For this review, take the finished solid that the model builds, in its own axes (mm). Face numbers are marked on the shaded views. A direction names the side the tool comes from. Give positions to 0.01 mm unless a question says otherwise; leave off trailing zeros. Write each loop counter-clockwise with the first axis right and the second up, starting at its lowest first coordinate (ties: lowest second). Pieces come first, ordered by that corner, then holes.
1) For P1, Ø3, axis at y = 3, z = 9, coming from the -X side; P2, Ø3, axis at x = 0, z = 8.03, coming from the +Y side, all flat-tipped, find the tip position at first contact; note any pin that passes through.
2) Wall thickness on line 1 along X through (y, z) = (1.1, 13); line 2 along X through (y, z) = (1.2, 14.5); line 3 along Y through (x, z) = (-1.5, 1.5): over which ranges is each line inside the solid? List them lowest first.
3) We need section B-B on y = 1.3. Give the number of separate pieces and of enclosed holes in the cut face, and give its area (3 significant figures).
4) We need section A-A on z = 6. Give the boundary of the cut face in (x, y), and give its area (3 significant figures).
5) Draft analysis for pull direction Z (two halves, no side actions). For the marked faces 6, 7, 8 and 9, state which applies: pulls with the +Z half, pulls with the -Z half, needs draft (parallel to the pull), parting line crosses it, or undercut.
6) Machinability: for the marked faces 1, 2, 3, 4 and 5, which of the approach directions +Z, -Z, +X, -X, +Y, -Y give a long, thin tool a straight path to every point of the face, cutting with its end or side? Answer none if there is none.
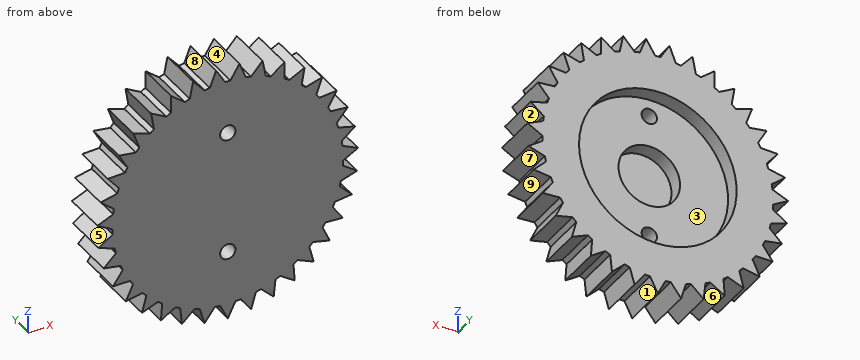
from build123d import *

# Parameters (mm, degrees)
SKETCH_1_R          = 15
EXTRUDE_1_DEPTH     = 6
EXTRUDE_2_DEPTH     = 6
SKETCH_3_R          = 1
CUT_EXTRUDE_1_DEPTH = 6
SKETCH_4_R          = 10.25
CUT_EXTRUDE_2_DEPTH = 2
SKETCH_5_R          = 4
CUT_EXTRUDE_3_DEPTH = 2


with BuildPart() as part:
    # 草图1 → 凸台-拉伸1 (new body)
    with BuildSketch(Plane(origin=(0, 0, 0), x_dir=(1, 0, 0), z_dir=(0, 1, 0))):
        Circle(SKETCH_1_R)
    extrude(amount=EXTRUDE_1_DEPTH)

    # 草图2 → 凸台-拉伸2 (add)
    with BuildSketch(Plane(origin=(0, 6, 0), x_dir=(1, 0, 0), z_dir=(0, 1, 0))):
        Polygon((0, 16.966629547), (-1, 14.966629547), (-1, 14.940773363), (1, 14.940773363), (1, 14.966629547), align=None)
        Polygon((3.656324486, 14.547552758), (3.029508687, 16.69396883), (1.688465309, 14.904666548), (1.683848509, 14.879225883), (3.651707686, 14.522112094), align=None)
        Polygon((6.195131695, 13.660905654), (5.961646472, 15.884750219), (4.322661954, 14.363655302), (4.313576741, 14.339447841), (6.186046483, 13.636698193), align=None)
        Polygon((8.534822274, 12.335185802), (8.702172035, 14.564982666), (6.817924686, 13.360984356), (6.804663068, 13.338788146), (8.521560655, 12.312989592), align=None)
        Polygon((10.600196642, 10.613002928), (11.163002628, 12.777084586), (9.09405371, 11.92888038), (9.077041925, 11.909408826), (10.583184857, 10.593531374), align=None)
        Polygon((12.324871968, 8.549709408), (13.265045131, 10.578520495), (11.077892365, 10.113372373), (11.057677186, 10.097251306), (12.30465679, 8.533588341), align=None)
        Polygon((13.653415769, 6.211621193), (14.94073817, 8.03995405), (12.705678444, 7.972812257), (12.682909604, 7.960559822), (13.630646929, 6.199368758), align=None)
        Polygon((14.543127552, 3.673886362), (16.13622359, 5.242976867), (13.925093563, 5.575999395), (13.900502871, 5.568009395), (14.51853686, 3.665896362), align=None)
        Polygon((14.96541125, 1.018069801), (16.813077508, 2.277486094), (14.696944718, 2.999969324), (14.671322539, 2.996498564), (14.939789071, 1.014599041), align=None)
        Polygon((14.906694317, -1.670468362), (16.94954528, -0.761204956), (14.996423977, 0.327517771), (14.970593829, 0.328677804), (14.880864168, -1.669308329), align=None)
        Polygon((14.368863963, -4.305316297), (16.541240721, -3.775430253), (14.813905831, -2.355460473), (14.788697915, -2.349706931), (14.343656047, -4.299562755), align=None)
        Polygon((13.369206498, -6.801787824), (15.601287075, -6.668310115), (14.155256562, -4.962732279), (14.131481082, -4.952570151), (13.345431019, -6.791625697), align=None)
        Polygon((11.939851737, -9.079644294), (14.159895226, -9.346865003), (13.0416457, -7.410497786), (13.02006682, -7.396253693), (11.918272857, -9.0654002), align=None)
        Polygon((10.126740316, -11.065673525), (12.263392693, -11.725003959), (11.508865614, -9.620083797), (11.490176897, -9.602215554), (10.1080516, -11.047805282), align=None)
        Polygon((7.98814713, -12.696042904), (9.972734629, -13.726291641), (9.606181119, -11.5204724), (9.590983235, -11.499554308), (7.972949246, -12.675124812), align=None)
        Polygon((5.592808322, -13.918351018), (7.361544668, -15.286405015), (7.394746058, -13.05058354), (7.38352748, -13.027287923), (5.581589744, -13.895055402), align=None)
        Polygon((3.017712053, -14.693311879), (4.513748605, -16.355200755), (4.945637774, -14.161238188), (4.938759077, -14.136313787), (3.010833355, -14.668387478), align=None)
        Polygon((0.345624035, -14.996017606), (1.520876947, -16.898326885), (2.337572623, -14.816738988), (2.335254893, -14.790986893), (0.343306305, -14.970265511), align=None)
        Polygon((-2.337572623, -14.816738988), (-1.520876947, -16.898326885), (-0.345624035, -14.996017606), (-0.343306305, -14.970265511), (-2.335254893, -14.790986893), align=None)
        Polygon((-4.945637774, -14.161238188), (-4.513748605, -16.355200755), (-3.017712053, -14.693311879), (-3.010833355, -14.668387478), (-4.938759077, -14.136313787), align=None)
        Polygon((-7.394746058, -13.05058354), (-7.361544668, -15.286405015), (-5.592808322, -13.918351018), (-5.581589744, -13.895055402), (-7.38352748, -13.027287923), align=None)
        Polygon((-9.606181119, -11.5204724), (-9.972734629, -13.726291641), (-7.98814713, -12.696042904), (-7.972949246, -12.675124812), (-9.590983235, -11.499554308), align=None)
        Polygon((-11.508865614, -9.620083797), (-12.263392693, -11.725003959), (-10.126740316, -11.065673525), (-10.108051599, -11.047805282), (-11.490176897, -9.602215554), align=None)
        Polygon((-13.0416457, -7.410497786), (-14.159895226, -9.346865003), (-11.939851737, -9.079644294), (-11.918272857, -9.0654002), (-13.02006682, -7.396253693), align=None)
        Polygon((-14.155256562, -4.962732279), (-15.601287075, -6.668310115), (-13.369206498, -6.801787824), (-13.345431019, -6.791625697), (-14.131481082, -4.952570151), align=None)
        Polygon((-14.813905831, -2.355460473), (-16.541240721, -3.775430253), (-14.368863963, -4.305316297), (-14.343656047, -4.299562755), (-14.788697915, -2.349706931), align=None)
        Polygon((-14.996423977, 0.327517771), (-16.94954528, -0.761204956), (-14.906694317, -1.670468362), (-14.880864168, -1.669308329), (-14.970593829, 0.328677804), align=None)
        Polygon((-14.696944718, 2.999969324), (-16.813077508, 2.277486094), (-14.96541125, 1.018069801), (-14.939789071, 1.014599041), (-14.671322539, 2.996498564), align=None)
        Polygon((-13.925093563, 5.575999395), (-16.13622359, 5.242976867), (-14.543127552, 3.673886362), (-14.51853686, 3.665896362), (-13.900502871, 5.568009395), align=None)
        Polygon((-12.705678444, 7.972812257), (-14.94073817, 8.03995405), (-13.653415769, 6.211621193), (-13.630646929, 6.199368758), (-12.682909604, 7.960559822), align=None)
        Polygon((-11.077892364, 10.113372373), (-13.265045131, 10.578520495), (-12.324871968, 8.549709408), (-12.30465679, 8.533588341), (-11.057677186, 10.097251306), align=None)
        Polygon((-9.09405371, 11.92888038), (-11.163002628, 12.777084586), (-10.600196642, 10.613002928), (-10.583184857, 10.593531374), (-9.077041925, 11.909408826), align=None)
        Polygon((-6.817924686, 13.360984356), (-8.702172035, 14.564982666), (-8.534822274, 12.335185802), (-8.521560655, 12.312989592), (-6.804663068, 13.338788146), align=None)
        Polygon((-4.322661954, 14.363655302), (-5.961646472, 15.884750219), (-6.195131695, 13.660905654), (-6.186046483, 13.636698193), (-4.313576741, 14.339447841), align=None)
        Polygon((-1.688465309, 14.904666548), (-3.029508687, 16.69396883), (-3.656324486, 14.547552758), (-3.651707686, 14.522112094), (-1.683848509, 14.879225883), align=None)
    extrude(amount=-EXTRUDE_2_DEPTH)

    # 草图3 → 切除-拉伸1 (cut)
    with BuildSketch(Plane(origin=(0, 6, 0), x_dir=(1, 0, 0), z_dir=(0, 1, 0))):
        with Locations((0, 7.966629547)):
            Circle(SKETCH_3_R)
        with Locations((0, -8.033370453)):
            Circle(SKETCH_3_R)
    extrude(amount=-CUT_EXTRUDE_1_DEPTH, mode=Mode.SUBTRACT)

    # 草图4 → 切除-拉伸2 (cut)
    with BuildSketch(Plane(origin=(0, 6, 0), x_dir=(1, 0, 0), z_dir=(0, 1, 0))):
        Circle(SKETCH_4_R)
    extrude(amount=-CUT_EXTRUDE_2_DEPTH, mode=Mode.SUBTRACT)

    # 草图5 → 切除-拉伸3 (cut)
    with BuildSketch(Plane(origin=(0, 4, 0), x_dir=(1, 0, 0), z_dir=(0, 1, 0))):
        Circle(SKETCH_5_R)
    extrude(amount=-CUT_EXTRUDE_3_DEPTH, mode=Mode.SUBTRACT)


solid = part.part
Results list:
1. P1: stops at x = -14.16
1. P2: stops at y = 4
2. line 1: x = -9.85 to -8.57, -7.48 to 7.48, 8.57 to 9.85
2. line 2: x = -7.37 to -6.34, -4.88 to 4.88, 6.34 to 7.37
2. line 3: y = 0 to 2
3. separate pieces: 1
3. enclosed holes: 2
3. area: 769 mm2
4. outline: (-15.03, 0) - (15.03, 0) - (15.03, 6) - (8.31, 6) - (8.31, 4) - (-8.31, 4) - (-8.31, 6) - (-15.03, 6) - close
4. area: 147 mm2
5. face 6: pulls with the -Z half
5. face 7: undercut
5. face 8: pulls with the +Z half
5. face 9: undercut
6. face 1: -Z, +Y, -Y
6. face 2: +X, +Y, -Y
6. face 3: +Y
6. face 4: +Z, +Y, -Y
6. face 5: -X, +Y, -Y
